The listing builds one solid part. Answer for the finished solid, in the listing's coordinates (mm). A direction names the side the tool comes from. Round coordinates to 2 decimals unless told otherwise and drop trailing zeros. Loops run counter-clockwise (first coordinate to the right, second up) from the corner with the lowest first, then second, coordinate; pieces in that order, holes last. Notation, with made-up numbers: (4.25, 2) -> (28.25, 2) arc R25 ccw to (28.25, 16) -> close; hole circle Ø11 at (0, 44.25). An arc over 180 degrees is marked (long way). Write each question's results on one line, items separated by ' | '. Start each with the question number.
from build123d import *

# Parameters (mm, degrees)
EXTRUDE_1_DEPTH     = 13
SKETCH_3_R          = 4.25
CUT_EXTRUDE_1_DEPTH = 67.580778007


with BuildPart() as part:
    # 草图1 → 凸台-拉伸1 (new, symmetric)
    with BuildSketch(Plane.XY):
        Polygon((0, 0), (50, 0), (50, 50), (42, 50), (42, 29.242640687), (20.757359313, 8), (0, 8), align=None)
        with BuildLine():
            Line((37.061279898, 14.352933665), (35.340960992, 16.07325257))
            ThreePointArc((35.340960992, 16.07325257), (39.856939547, 16.192314452), (42.15, 12.3))
            Line((42.15, 12.3), (45, 12.3))
            Line((45, 12.3), (45, 23.171572875))
            ThreePointArc((45, 23.171572875), (43.765366865, 25.01933194), (41.585786438, 24.585786438))
            Line((41.585786438, 24.585786438), (25.414213562, 8.414213562))
            ThreePointArc((25.414213562, 8.414213562), (24.98066806, 6.234633135), (26.828427125, 5))
            Line((26.828427125, 5), (37.7, 5))
            Line((37.7, 5), (37.7, 7.85))
            ThreePointArc((37.7, 7.85), (33.807685548, 10.143060453), (33.92674743, 14.659039008))
            Line((33.92674743, 14.659039008), (35.647066335, 12.938720102))
            ThreePointArc((35.647066335, 12.938720102), (39.22027958, 10.77972042), (37.061279898, 14.352933665))
        make_face(mode=Mode.SUBTRACT)
    extrude(amount=EXTRUDE_1_DEPTH, both=True)

    # 草图3 → 切除-拉伸1 (cut, through all)
    with BuildSketch(Plane(origin=(0, 8, 0), x_dir=(1, 0, 0), z_dir=(0, 1, 0))):
        with Locations(Location((10, 0, 0), (0, 0, 270))):
            Circle(SKETCH_3_R)
    cut_extrude_1 = extrude(amount=-CUT_EXTRUDE_1_DEPTH, mode=Mode.SUBTRACT)

    # 镜向1: 切除-拉伸1 across plane
    add(cut_extrude_1.mirror(Plane(origin=(25, 25, 0), x_dir=(0, 0, 1), z_dir=(-0.7071067811865489, -0.7071067811865462, 0))), mode=Mode.SUBTRACT)


solid = part.part
Item 1: The part is cut by section C-C, the plane x = 10. Give the vertices of the cut face in (y, z).
Item 2: Straight lines are drawn through the part: L1, parallel to X at y = 16, z = -6; L2, parallel to X at y = 11, z = 11.75; L3, parallel to Y at x = 34, z = -3. For each, find the intervals that lie inside material, in ascending order. Write a range as [from, to].
Item 3: For faces 1 (the flat face through (42, 35, 0)), 2 (the flat face through (32, 5, 0)), 3 (the cylindrical face through (5.85, 4.06, -0.92)), determine the directions among +Z, -Z, +X, -X, +Y, -Y from which every point of the face is accessible in a straight line to the end or side of a thin tool.
Item 4: Each of these flat-tipped pins is pushed along its axis until it touches: pin 1 Ø10 at (x, z) = (10, 0) entering from +Y; pin 2 Ø8.5 at (x, z) = (30.5, 4.5) entering from +Y; pin 3 Ø6 at (x, z) = (31, -5.5) entering from +Y. Where does it stop, or does it pass through?
Item 5: Determine the mould class of faces 4 (the flat face through (46, 50, 0)), 5 (the flat face through (50, 25, 0)), 6 (the cylindrical face through (24.968, 6.265, 0.182)), 7 (the flat face through (0, 4, 0)) for opening direction X: +X half, -X half, draft (parallel to the pull), parting line (faces both ways), or undercut.
Item 6: The part is cut by section B-B, the plane y = 40. Give the vertices of the cut face in (x, z), plus the area to 3 significant figures.
Item 7: The part is cut by section D-D, the plane z = -9.5. Give the vertices of the cut face in (x, y), plus the area to 3 significant figures.
Item 8: The part is cut by section A-A, the plane z = -2. Give the vertices of the cut face in (x, y).
Report:
1) outline: (0, -13) -> (8, -13) -> (8, -4.25) -> (0, -4.25) -> close; (0, 4.25) -> (8, 4.25) -> (8, 13) -> (0, 13) -> close
2) L1: x = [28.76, 33], [35.41, 40.17], [45, 50] | L2: x = [23.76, 28], [33.44, 35.99], [39.41, 50] | L3: y = [0, 5], [9.83, 14.59], [17, 21.24]
3) face 1: +Z, -Z, -X, +Y | face 2: +Z, -Z | face 3: +Y, -Y
4) pin 1: stops at y = 8 | pin 2: stops at y = 21.99 | pin 3: stops at y = 21.24
5) face 4: draft | face 5: +X half | face 6: undercut | face 7: -X half
6) outline: (42, -13) -> (50, -13) -> (50, -4.25) -> (42, -4.25) -> close; (42, 4.25) -> (50, 4.25) -> (50, 13) -> (42, 13) -> close | area: 140 mm2
7) outline: (0, 0) -> (50, 0) -> (50, 50) -> (42, 50) -> (42, 29.24) -> (20.76, 8) -> (0, 8) -> close; hole (25.41, 8.41) arc R2 ccw to (26.83, 5) -> (37.7, 5) -> (37.7, 7.85) arc R4.45 cw to (33.93, 14.66) -> (35.65, 12.94) arc R2.15 ccw (long way) to (37.06, 14.35) -> (35.34, 16.07) arc R4.45 cw to (42.15, 12.3) -> (45, 12.3) -> (45, 23.17) arc R2 ccw to (41.59, 24.59) -> close | area: 788 mm2
8) outline: (0, 0) -> (6.25, 0) -> (6.25, 8) -> (0, 8) -> close; (13.75, 0) -> (50, 0) -> (50, 36.25) -> (42, 36.25) -> (42, 29.24) -> (20.76, 8) -> (13.75, 8) -> close; (42, 43.75) -> (50, 43.75) -> (50, 50) -> (42, 50) -> close; hole (25.41, 8.41) arc R2 ccw to (26.83, 5) -> (37.7, 5) -> (37.7, 7.85) arc R4.45 cw to (33.93, 14.66) -> (35.65, 12.94) arc R2.15 ccw (long way) to (37.06, 14.35) -> (35.34, 16.07) arc R4.45 cw to (42.15, 12.3) -> (45, 12.3) -> (45, 23.17) arc R2 ccw to (41.59, 24.59) -> close
